from build123d import *

# Parameters (mm, degrees)
SKETCH1_W                  = 88.9
SKETCH1_H                  = 88.9
EXTRUDE1_DEPTH             = 12.7
EXTRUDE2_DEPTH             = 127.363404513
EXTRUDE9_DEPTH             = 127.363404513
SKETCH4_W                  = 76.2
SKETCH4_H                  = 279.4
EXTRUDE3_DEPTH             = 12.7
EXTRUDE7_DEPTH             = 622.292826593
EXTRUDE6_REACH             = 742.115
EXTRUDE6_START             = 127
SKETCH7_R                  = 25.4
SKETCH7_R_2                = 12.7
EXTRUDE6_DIRECTION_2_REACH = 742.115
EXTRUDE10_DEPTH            = 676.899389977
SKETCH9_W                  = 7.874
SKETCH9_H                  = 127
EXTRUDE8_DEPTH             = 622.292826593


with BuildPart() as part:
    # Sketch1 → Extrude1 (new body)
    with BuildSketch(Plane(origin=(0, 0, 0), x_dir=(1, 0, 0), z_dir=(0, 1, 0))):
        with Locations((-44.45, 44.45)):
            Rectangle(SKETCH1_W, SKETCH1_H)
    extrude(amount=EXTRUDE1_DEPTH)

    # Sketch2 → Extrude2 (cut, through all)
    with BuildSketch(Plane(origin=(0, 12.7, 0), x_dir=(1, 0, 0), z_dir=(0, 1, 0))):
        with BuildLine():
            Line((-19.05, 15.748), (-19.05, 22.098))
            ThreePointArc((-19.05, 22.098), (-12.7, 28.448), (-6.35, 22.098))
            Line((-6.35, 22.098), (-6.35, 15.748))
            ThreePointArc((-6.35, 15.748), (-12.7, 9.398), (-19.05, 15.748))
        make_face()
        with BuildLine():
            Line((-19.05, 62.484), (-19.05, 68.834))
            ThreePointArc((-19.05, 68.834), (-12.7, 75.184), (-6.35, 68.834))
            Line((-6.35, 68.834), (-6.35, 62.484))
            ThreePointArc((-6.35, 62.484), (-12.7, 56.134), (-19.05, 62.484))
        make_face()
        with BuildLine():
            Line((-85.725, 68.834), (-85.725, 75.184))
            ThreePointArc((-85.725, 75.184), (-79.375, 81.534), (-73.025, 75.184))
            Line((-73.025, 75.184), (-73.025, 68.834))
            ThreePointArc((-73.025, 68.834), (-79.375, 62.484), (-85.725, 68.834))
        make_face()
    extrude(amount=-EXTRUDE2_DEPTH, mode=Mode.SUBTRACT)

    # Sketch10 → Extrude9 (cut, through all)
    with BuildSketch(Plane.XZ):
        Polygon((-88.9, -49.022), (-39.878, 0), (-88.9, 0), align=None)
    extrude(amount=-EXTRUDE9_DEPTH, mode=Mode.SUBTRACT)



with BuildPart() as body_2:
    # Sketch4 → Extrude3 (new body)
    with BuildSketch(Plane(origin=(0, 0, 42.926), x_dir=(-1, 0, 0), z_dir=(0, 0, -1))):
        with Locations((-49.784, 463.55)):
            Rectangle(SKETCH4_W, SKETCH4_H)
    extrude(amount=EXTRUDE3_DEPTH)

    # Sketch8 → Extrude7 (cut, through all)
    with BuildSketch(Plane(origin=(0, 0, 30.226), x_dir=(-1, 0, 0), z_dir=(0, 0, -1))):
        with BuildLine():
            Line((-24.384, 587.375), (-24.384, 581.025))
            ThreePointArc((-24.384, 581.025), (-30.734, 574.675), (-37.084, 581.025))
            Line((-37.084, 581.025), (-37.084, 587.375))
            ThreePointArc((-37.084, 587.375), (-30.734, 593.725), (-24.384, 587.375))
        make_face()
        with BuildLine():
            Line((-24.384, 555.625), (-24.384, 549.275))
            ThreePointArc((-24.384, 549.275), (-30.734, 542.925), (-37.084, 549.275))
            Line((-37.084, 549.275), (-37.084, 555.625))
            ThreePointArc((-37.084, 555.625), (-30.734, 561.975), (-24.384, 555.625))
        make_face()
        with BuildLine():
            Line((-64.0842, 346.075), (-64.0842, 339.725))
            ThreePointArc((-64.0842, 339.725), (-70.4342, 333.375), (-76.7842, 339.725))
            Line((-76.7842, 339.725), (-76.7842, 346.075))
            ThreePointArc((-76.7842, 346.075), (-70.4342, 352.425), (-64.0842, 346.075))
        make_face()
    extrude(amount=-EXTRUDE7_DEPTH, mode=Mode.SUBTRACT)


with BuildPart() as part_1:
    add(part.part)

    add(body_2.part)  # Extrude6 merges body 2
    # Extrude6: up to this plane
    extrude6_end = Plane(origin=(11.684, 323.85, 30.226), z_dir=(0, 0, 1))
    # Sketch7 → Extrude6 (add, up to the surface)
    with BuildSketch(Plane(origin=(-44.958, 12.7, -54.61), x_dir=(-0.9783852357673664, 0.18254912655536365, 0.09715012519965675), z_dir=(0.1967453547942853, 0.9663814656142476, 0.16552379975136336)).offset(EXTRUDE6_START), mode=Mode.PRIVATE) as extrude6_sk1:
        with Locations(Location((0, 0, 0), (0, 0, 189.444307403))):
            Circle(SKETCH7_R)
        with Locations(Location((0, 0, 0), (0, 0, 84.346682726))):
            Circle(SKETCH7_R_2, mode=Mode.SUBTRACT)
    extrude6_tool1 = split(extrude(extrude6_sk1.sketch, amount=EXTRUDE6_REACH, mode=Mode.PRIVATE), bisect_by=extrude6_end, keep=Keep.BOTH, mode=Mode.PRIVATE)
    add(extrude6_tool1.solids().sort_by_distance((-43.534266, 139.141689, -27.248481))[0])

    # Extrude6 direction 2: up to this plane
    extrude6_direction_2_end = Plane(origin=(0, 12.7, -88.9), z_dir=(0, 1, 0))
    # Sketch7 → Extrude6 direction 2 (add, up to the surface)
    with BuildSketch(Plane(origin=(-44.958, 12.7, -54.61), x_dir=(-0.9783852357673664, 0.18254912655536365, 0.09715012519965675), z_dir=(0.1967453547942853, 0.9663814656142476, 0.16552379975136336)).offset(EXTRUDE6_START), mode=Mode.PRIVATE) as extrude6_direction_2_sk1:
        with Locations(Location((0, 0, 0), (0, 0, 189.444307403))):
            Circle(SKETCH7_R)
        with Locations(Location((0, 0, 0), (0, 0, 84.346682726))):
            Circle(SKETCH7_R_2, mode=Mode.SUBTRACT)
    extrude6_direction_2_tool1 = split(extrude(extrude6_direction_2_sk1.sketch, amount=-EXTRUDE6_DIRECTION_2_REACH, mode=Mode.PRIVATE), bisect_by=extrude6_direction_2_end, keep=Keep.BOTH, mode=Mode.PRIVATE)
    add(extrude6_direction_2_tool1.solids().sort_by_distance((-43.534266, 139.141689, -27.248481))[0])

    # Sketch11 → Extrude10 (cut, through all)
    with BuildSketch(Plane.XY.offset(30.226)):
        with BuildLine():
            Line((54.665648122, 603.25), (87.884, 603.25))
            Line((87.884, 603.25), (87.884, 542.273095972))
            add(Edge.make_bspline(
                [(87.884, 542.273095972), (134.728854914, 839.694203258), (54.665648122, 603.25)],
                knots=[1.834299587, 1.834299587, 1.834299587, 4.060538938, 4.060538938, 4.060538938], degree=2, weights=[1, 0.441865068, 1]))
        make_face()
    extrude(amount=-EXTRUDE10_DEPTH, mode=Mode.SUBTRACT)

    # Sketch9 → Extrude8 (cut, through all)
    with BuildSketch(Plane(origin=(0, 0, 30.226), x_dir=(-1, 0, 0), z_dir=(0, 0, -1))):
        with Locations((-83.947, 387.35)):
            Rectangle(SKETCH9_W, SKETCH9_H)
    extrude(amount=-EXTRUDE8_DEPTH, mode=Mode.SUBTRACT)


solid = part_1.part
CAD build for the part. Positions are in the model's coordinates, mm. A direction names the side the tool comes from. Round coordinates to 2 decimals unless told otherwise and drop trailing zeros. Put each result on its own line as item: value.
1. Wall check: line 1 (X direction, y = 453, z = 37); line 2 (Y direction, x = -71, z = -43); line 3 (Z direction, x = 6, y = 206). Give the ranges that are in metal, low to high.
Geometry check:
line 1: 11.68 to 87.88
line 2: 0 to 12.7
line 3: -44.14 to -26.85, -15.38 to 1.92
2. Slice it at A-A on x = -12.7. Give the number of separate pieces and of enclosed holes in the cut face, and give its area (3 significant figures).
Geometry check:
separate pieces: 4
enclosed holes: 1
area: 8,370 mm²
3. Two-plate mould, pull along Z, no slides. Class faces 6 (the cylindrical face through (70.574, 352.423, 36.487)), 7 (the flat face through (67, 434, 30.226)), 8 (the flat face through (50, 466, 42.926)): released by +Z, released by -Z, zero draft, split by the parting line, or undercut.
Geometry check:
face 6: zero draft
face 7: undercut
face 8: released by +Z
4. 3-axis set-ups, long thin cutter, end or side, ignore diameter. For faces 1 (the cylindrical face through (-12.56, 6.439, -56.136)), 2 (the flat face through (11.684, 462, 37)), 3 (the cylindrical face through (70.295, 333.377, 36.487)), 4 (the cylindrical face through (-12.84, 6.439, -75.182)), 5 (the flat face through (-45, 12.7, -55)): which of +Z, -Z, +X, -X, +Y, -Y reach the whole face in a straight line?
Geometry check:
face 1: -Y
face 2: +Z, -X, +Y, -Y
face 3: +Z, -Z
face 4: +Y, -Y
face 5: none
5. Pin check, flat tips, straight feed: P1, Ø10, axis at y = 8.5, z = -27.5, coming from the +X side; P2, Ø8.5, axis at x = 85.5, z = 36.5, coming from the -Y side; P3, Ø10, axis at x = 55, z = 37, coming from the -Y side. Stop position of each tip, or through.
Geometry check:
P1: x = 0
P2: y = 450.85
P3: y = 323.85
